Source: CAD feature listing. Evaluate the final solid. Frame: model axes, mm. A direction names the side the tool comes from. Give positions to 0.01 mm unless a question says otherwise; leave off trailing zeros. Loops run counter-clockwise (first coordinate to the right, second up) from the corner with the lowest first, then second, coordinate; pieces in that order, holes last. Notation, with made-up numbers: (70.5, 89) -> (108.5, 89) arc R15 ccw to (108.5, 101) -> close; hole circle Ø11 at (0, 66.25). An arc over 180 degrees is marked (long way). Return JSON: item names as keys, results as strings. Group by question number.
(1) Draft query along Z for faces 4 (the face through (-0.83, 130.07, -2.883)), 5 (the face through (20.03, 15.78, -6.31)), 6 (the face through (6.81, 110.93, -16.35)). Return one class per face: released by +Z, released by -Z, zero draft, split by the parting line, or undercut.
(2) Cut plane D-D on y = 38.5. Return loops of the section in (x, z).
(3) Access query for faces 1 (the face through (-6.01, 113.52, 14.13)), 2 (the face through (0, 135, 0)), 3 (the face through (-7.493, -2.465, 0.33)). Directions: +Z, -Z, +X, -X, +Y, -Y. A direction counts if a zero-diameter tool reaches every point of the face in a straight line with its end or side. Return the directions, or none.
(4) Cut plane A-A on z = 0. Return loops of the section in (x, y).
(5) Pin query (flat end, axial travel): pin 1 (4 mm diameter, centred on x = -1.5, y = 69, fed in from +Z); pin 2 (4 mm diameter, centred on x = -4, z = -9, fed in from -Y); pin 3 (6 mm diameter, centred on y = 120, z = -16.5, fed in from +X); pin 4 (10 mm diameter, centred on x = -15, y = 95.5, fed in from +Z). Return the tip coordinate at first contact, or that it passes through.
(6) Cut plane B-B on y = 7.5. Return loops of the section in (x, z).
(7) Ray query, line 1 (Z direction, x = 0.5, y = 86); line 2 (Y direction, x = -12.5, z = -2); line 3 (X direction, y = 106.5, z = 1). Return the intervals inside material, ascending. Write a range as from..to.
```python
from build123d import *

# Parameters (mm, degrees)
SKETCH1_R           = 21
BOSS_EXTRUDE1_DEPTH = 72
SKETCH3_R           = 23
SKETCH3_R_2         = 21
BOSS_EXTRUDE2_DEPTH = 30
SKETCH4_R           = 20.85
BOSS_EXTRUDE3_DEPTH = 43
SKETCH5_R           = 13
BOSS_EXTRUDE4_DEPTH = 2
SKETCH6_R           = 4
BOSS_EXTRUDE5_DEPTH = 18
SKETCH8_R           = 7.5
BOSS_EXTRUDE6_DEPTH = 5
CIRPATTERN1_COUNT   = 4
CUT_EXTRUDE1_DEPTH  = 10


with BuildPart() as part:
    # Sketch1 → Boss-Extrude1 (new body)
    with BuildSketch(Plane(origin=(0, 0, 0), x_dir=(1, 0, 0), z_dir=(0, 1, 0))):
        Circle(SKETCH1_R)
    extrude(amount=BOSS_EXTRUDE1_DEPTH)

    # Sketch3 → Boss-Extrude2 (add)
    with BuildSketch(Plane(origin=(0, 62, 0), x_dir=(1, 0, 0), z_dir=(0, 1, 0))):
        Circle(SKETCH3_R)
        Circle(SKETCH3_R_2, mode=Mode.SUBTRACT)
    extrude(amount=-BOSS_EXTRUDE2_DEPTH)

    # Sketch4 → Boss-Extrude3 (add)
    with BuildSketch(Plane(origin=(0, 72, 0), x_dir=(1, 0, 0), z_dir=(0, 1, 0))):
        Circle(SKETCH4_R)
    extrude(amount=BOSS_EXTRUDE3_DEPTH)

    # Sketch5 → Boss-Extrude4 (add)
    with BuildSketch(Plane(origin=(0, 115, 0), x_dir=(1, 0, 0), z_dir=(0, 1, 0))):
        Circle(SKETCH5_R)
    extrude(amount=BOSS_EXTRUDE4_DEPTH)

    # Sketch6 → Boss-Extrude5 (add)
    with BuildSketch(Plane(origin=(0, 117, 0), x_dir=(1, 0, 0), z_dir=(0, 1, 0))):
        Circle(SKETCH6_R)
    extrude(amount=BOSS_EXTRUDE5_DEPTH)

    # Sketch8 → Boss-Extrude6 (add)
    with BuildSketch(Plane.XZ):
        Circle(SKETCH8_R)
    extrude(amount=BOSS_EXTRUDE6_DEPTH)

    # Sketch14 → CSK for M4 Flat Head Machine Screw1 (revolve, cut)
    with BuildSketch(Plane(origin=(-16.036289765, 117, -7.00624083), x_dir=(0, 0, 1), z_dir=(1, 0, 0))):
        Polygon((0, 0), (0, 6.291850331), (2.15, 5), (2.15, 0.6), (2.75, 0), align=None)
    csk_for_m4_flat_head_machine_screw1 = revolve(axis=Axis((-16.036289765, 123.35, -7.00624083), (0, -1, 0)), mode=Mode.SUBTRACT)

    # CirPattern1: CSK for M4 Flat Head Machine Screw1 ×4 about axis
    cirpattern1_axis = Axis((0, 0, 0), (0, 1, 0))
    for i in range(1, CIRPATTERN1_COUNT):
        add(csk_for_m4_flat_head_machine_screw1.rotate(cirpattern1_axis, i * 360 / CIRPATTERN1_COUNT), mode=Mode.SUBTRACT)

    # Sketch17 → Cut-Extrude1 (cut)
    with BuildSketch(Plane(origin=(0, 135, 0), x_dir=(1, 0, 0), z_dir=(0, 1, 0))):
        with BuildLine():
            Line((-3.345642255, 2.192413717), (1.757012768, 3.593453233))
            ThreePointArc((1.757012768, 3.593453233), (-1.059086325, 3.857244633), (-3.345642255, 2.192413717))
        make_face()
    extrude(amount=-CUT_EXTRUDE1_DEPTH, mode=Mode.SUBTRACT)


solid = part.part
```
Answers:
{
 "1": {"face 4": "released by -Z", "face 5": "split by the parting line", "face 6": "undercut"},
 "2": {"outline": "circle Ø46 at (0, 0)"},
 "3": {"face 1": "+Y", "face 2": "+Z, -Z, +X, -X, +Y", "face 3": "-Y"},
 "4": {"outline": "(-23, 32) -> (-21, 32) -> (-21, 0) -> (-7.5, 0) -> (-7.5, -5) -> (7.5, -5) -> (7.5, 0) -> (21, 0) -> (21, 32) -> (23, 32) -> (23, 62) -> (21, 62) -> (21, 72) -> (20.85, 72) -> (20.85, 115) -> (13, 115) -> (13, 117) -> (4, 117) -> (4, 135) -> (-4, 135) -> (-4, 117) -> (-13, 117) -> (-13, 115) -> (-20.85, 115) -> (-20.85, 72) -> (-21, 72) -> (-21, 62) -> (-23, 62) -> close"},
 "5": {"pin 1": "z = 21", "pin 2": "y = 0", "pin 3": "through", "pin 4": "z = 18.3"},
 "6": {"outline": "circle Ø42 at (0, 0)"},
 "7": {"line 1": "-20.84..20.84", "line 2": "0..117", "line 3": "-20.83..20.83"}
}
